from build123d import *

# Parameters (mm, degrees)
CYLINDER005_R     = 5.25
CYLINDER005_DEPTH = 10
CYLINDER003_R     = 5.75
CYLINDER003_DEPTH = 10
CYLINDER004_R     = 7
CYLINDER004_DEPTH = 7


with BuildPart() as holderlenssmall:
    # Cylinder005 → Cylinder005 (new body)
    with BuildSketch(Plane.XY):
        Circle(CYLINDER005_R)
    extrude(amount=CYLINDER005_DEPTH)


with BuildPart() as holderlens:
    # Cylinder003 → Cylinder003 (new body)
    with BuildSketch(Plane.XY.offset(1)):
        Circle(CYLINDER003_R)
    extrude(amount=CYLINDER003_DEPTH)


with BuildPart() as lensholder01:
    # Cylinder004 → Cylinder004 (new body)
    with BuildSketch(Plane.XY):
        Circle(CYLINDER004_R)
    extrude(amount=CYLINDER004_DEPTH)

    # Cut003: cut HolderLens
    add(holderlens.part, mode=Mode.SUBTRACT)

    # Cut004: cut HolderLensSmall
    add(holderlenssmall.part, mode=Mode.SUBTRACT)


solid = lensholder01.part
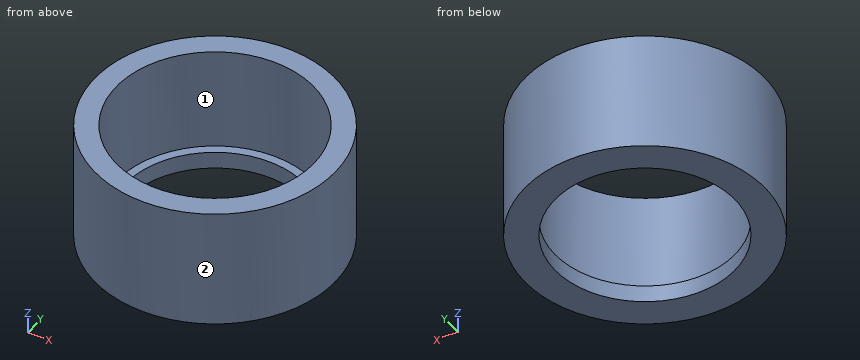
CAD build for the part. Positions are in the model's coordinates, mm. Face numbers are marked on the shaded views. A direction names the side the tool comes from. Round coordinates to 2 decimals unless told otherwise and drop trailing zeros. Order: outer loops, then holes, each group sorted by start corner. A loop starts at its lowest first (then second) coordinate and runs counter-clockwise, first axis right, second up. Notation, with made-up numbers: (-31.75, 55.5) -> (-26.75, 55.5) arc R12 cw to (-26.75, 62.5) -> close; hole circle Ø10 at (-22, 75.5). An arc over 180 degrees is marked (long way). Write each question's results on one line, items separated by ' | '.
1. Cut at A-A (y = 0). Give the cut face in (x, z), plus the area to 3 significant figures.
Findings below:
outline: (-7, 0) -> (-5.25, 0) -> (-5.25, 1) -> (-5.75, 1) -> (-5.75, 7) -> (-7, 7) -> close; (5.25, 0) -> (7, 0) -> (7, 7) -> (5.75, 7) -> (5.75, 1) -> (5.25, 1) -> close | area: 18.5 mm²
2. 3-axis set-ups, long thin cutter, end or side, ignore diameter. For the marked faces 1 and 2: which of +Z, -Z, +X, -X, +Y, -Y reach the whole face in a straight line?
Findings below:
face 1: +Z | face 2: +Z, -Z
3. Flat gauge pins, fed straight in: P1, Ø1, axis at y = 3, z = 1, coming from the +X side; P2, Ø1, axis at y = -3, z = 6, coming from the -X side; P3, Ø1, axis at y = -2.5, z = 4, coming from the -X side. Where does each tip first touch, or does it go through?
Findings below:
P1: stops at x = 6.54 | P2: stops at x = -6.54 | P3: stops at x = -6.71
4. Wall check: line 1 along Y through (x, z) = (0, 0.35); line 2 along Y through (x, z) = (0, 2.5); line 3 along X through (y, z) = (1, 2). Give the ranges that are in metal, low to high. Write a range as [from, to].
Findings below:
line 1: y = [-7, -5.25], [5.25, 7] | line 2: y = [-7, -5.75], [5.75, 7] | line 3: x = [-6.93, -5.66], [5.66, 6.93]
5. Cut at C-C (z = 1.25). Give the cut face in (x, y).
Findings below:
outline: circle Ø14 at (0, 0); hole circle Ø11.5 at (0, 0)
